Design review of the part built by this model. Coordinates are the model's own, in mm. Face numbers are marked on the shaded views. A direction names the side the tool comes from. Round coordinates to 2 decimals unless told otherwise and drop trailing zeros. Loops run counter-clockwise (first coordinate to the right, second up) from the corner with the lowest first, then second, coordinate; pieces in that order, holes last. Notation, with made-up numbers: (52.5, -6) - (77.5, -6) arc R23 ccw to (77.5, 18) - close; hole circle Ø6 at (-31, 46). An arc over 180 degrees is marked (long way). Answer as CSV lines item,"result". Start each with the question number.
(1) Consider section A-A (z = 1.5). Give the boundary of the cut face in (x, y).
(2) For P1, Ø6.5, axis at x = -5, y = 4, coming from the -Z side; P2, Ø2.5, axis at x = -1.5, z = 1.5, coming from the -Y side; P3, Ø1.5, axis at x = 2, z = 1.5, coming from the +Y side; P4, Ø2.5, axis at y = -2.5, z = 1.5, coming from the +X side, all flat-tipped, find the tip position at first contact; note any pin that passes through.
(3) Wall thickness on L1, parallel to Z at x = 4.5, y = 7; L2, parallel to Y at x = -1.25, z = 1; L3, parallel to Z at x = -3.5, y = 0.25: over which ranges is each line inside the solid? List them lowest first.
(4) For the marked faces 1, 2 and 3, list the 3-axis set-ups (+Z, -Z, +X, -X, +Y, -Y) from which the entire face can be reached by the end or side of a thin tool; tool diameter is ignored.
(5) Consider section D-D (z = 4.25). Give the boundary of the cut face in (x, y).
(6) Consider section B-B (x = 0). Give the boundary of the cut face in (y, z), and give its area (3 significant figures).
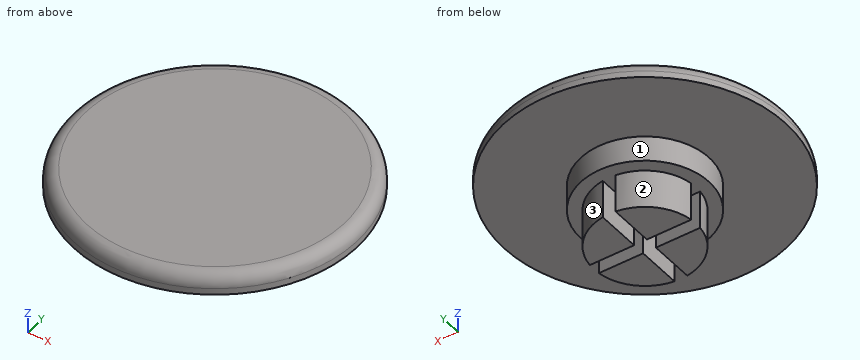
from build123d import *

# Parameters (mm, degrees)
F3_DEPTH = 3
F4_R     = 1


with BuildPart() as f1:
    # F0 (on Front) → F1 (revolve)
    with BuildSketch(Plane.XZ):
        Polygon((0, 6.5), (0, 0), (4, 0), (4, 3), (5, 3), (5, 5), (11, 5), (11, 6.5), align=None)
    revolve(axis=Axis((0, 0, 5.302473), (0, 0, 1)))

    # F2 (on face) → F3 (cut, through all)
    with BuildSketch(Plane(origin=(0, 0, 0), x_dir=(1, 0, 0), z_dir=(0, 0, -1))):
        Polygon((-0.5, -6.403249), (0.5, -6.403249), (0.5, -0.5), (5.621079, -0.5), (5.621079, 0.5), (0.5, 0.5), (0.5, 6.403249), (-0.5, 6.403249), (-0.5, 0.5), (-5.621079, 0.5), (-5.621079, -0.5), (-0.5, -0.5), align=None)
    extrude(amount=-F3_DEPTH, mode=Mode.SUBTRACT)

    # F4
    f4_edges = [f1.edges().sort_by_distance(p)[0] for p in [
        (-11, 0, 6.5),
    ]]
    fillet(f4_edges, radius=F4_R)


solid = f1.part
Determined:
1,outline,"(-3.97, -0.5) arc R4 ccw to (-0.5, -3.97) - (-0.5, -0.5) - close; (-3.97, 0.5) - (-0.5, 0.5) - (-0.5, 3.97) arc R4 ccw to start; (0.5, -3.97) arc R4 ccw to (3.97, -0.5) - (0.5, -0.5) - close; (0.5, 0.5) - (3.97, 0.5) arc R4 ccw to (0.5, 3.97) - close"
2,P1,"stops at z = 0"
2,P2,"stops at y = -3.97"
2,P3,"stops at y = 3.8"
2,P4,"stops at x = 3.8"
3,L1,"z = 5 to 6.5"
3,L2,"y = -3.8 to -0.5, 0.5 to 3.8"
3,L3,"z = 3 to 6.5"
4,face 1,"-Z"
4,face 2,"-Z, -X, +Y"
4,face 3,"-Z, +X, +Y"
5,outline,"circle Ø10 at (0, 0)"
6,outline,"(-11, 5) - (-5, 5) - (-5, 3) - (5, 3) - (5, 5) - (11, 5) - (11, 5.5) arc R1 ccw to (10, 6.5) - (-10, 6.5) arc R1 ccw to (-11, 5.5) - close"
6,area,"52.6 mm^2"
